from build123d import *

# Parameters (mm, degrees)
SKETCH1_W           = 40.1
SKETCH1_H           = 28.6
SKETCH1_W_2         = 36.5
SKETCH1_H_2         = 25
BOSS_EXTRUDE1_DEPTH = 8
SKETCH2_W           = 40.1
SKETCH2_H           = 28.6
SKETCH2_W_2         = 31
SKETCH2_H_2         = 23
BOSS_EXTRUDE2_DEPTH = 2
FILLET1_R           = 4
FILLET4_R           = 3
FILLET5_R           = 3
CUT_EXTRUDE1_REACH  = 45.732


with BuildPart() as part:
    # Sketch1 → Boss-Extrude1 (new body)
    with BuildSketch(Plane(origin=(0, 0, 0), x_dir=(1, 0, 0), z_dir=(0, 1, 0))):
        Rectangle(SKETCH1_W, SKETCH1_H)
        Rectangle(SKETCH1_W_2, SKETCH1_H_2, mode=Mode.SUBTRACT)
    extrude(amount=BOSS_EXTRUDE1_DEPTH)

    # Sketch2 → Boss-Extrude2 (add)
    with BuildSketch(Plane(origin=(0, 8, 0), x_dir=(1, 0, 0), z_dir=(0, 1, 0))):
        Rectangle(SKETCH2_W, SKETCH2_H)
        with Locations((-1.25, 0)):
            Rectangle(SKETCH2_W_2, SKETCH2_H_2, mode=Mode.SUBTRACT)
    extrude(amount=BOSS_EXTRUDE2_DEPTH)

    # Fillet1
    fillet1_edges = [part.edges().sort_by_distance(p)[0] for p in [
        (20.05, 5, 14.3),
        (-20.05, 5, 14.3),
        (-20.05, 5, -14.3),
        (20.05, 5, -14.3),
    ]]
    fillet(fillet1_edges, radius=FILLET1_R)

    # Fillet4
    # the kernel refuses this fillet: 3 mm, written as the material it takes off along each edge
    with BuildSketch(Plane(origin=(-20.05, 10, 10.3), x_dir=(1, 0, 0), z_dir=(0, 0, -1)), Plane(origin=(20.05, 10, -10.3), x_dir=(-1, 0, 0), z_dir=(0, 0, 1))) as fillet4_piece_1:
        with BuildLine():
            CenterArc((FILLET4_R, FILLET4_R), FILLET4_R, 180, 90)
            Line((0, FILLET4_R), (0, 0))
            Line((0, 0), (FILLET4_R, 0))
        make_face()
    extrude(amount=20.6, mode=Mode.SUBTRACT)
    with BuildSketch(Plane(origin=(-16.05, 10, -10.3), x_dir=(0, 0, -1), z_dir=(1, 0, 0))) as fillet4_piece_2:
        with BuildLine():
            CenterArc((4 - FILLET4_R, -FILLET4_R), FILLET4_R, 0, 90)
            Line((4, -FILLET4_R), (4, 0))
            Line((4, 0), (4 - FILLET4_R, 0))
        make_face()
    revolve(axis=Axis((-16.05, 10, -10.3), (0, 1, 0)), revolution_arc=90, mode=Mode.SUBTRACT)
    with BuildSketch(Plane(origin=(-16.05, 10, -14.3), x_dir=(0, 0, 1), z_dir=(1, 0, 0))) as fillet4_piece_3:
        with BuildLine():
            CenterArc((FILLET4_R, FILLET4_R), FILLET4_R, 180, 90)
            Line((0, FILLET4_R), (0, 0))
            Line((0, 0), (FILLET4_R, 0))
        make_face()
    extrude(amount=32.1, mode=Mode.SUBTRACT)
    with BuildSketch(Plane(origin=(16.05, 10, -10.3), x_dir=(0, 0, -1), z_dir=(-1, 0, 0))) as fillet4_piece_4:
        with BuildLine():
            CenterArc((4 - FILLET4_R, FILLET4_R), FILLET4_R, 270, 90)
            Line((4, FILLET4_R), (4, 0))
            Line((4, 0), (4 - FILLET4_R, 0))
        make_face()
    revolve(axis=Axis((16.05, 10, -10.3), (0, -1, 0)), revolution_arc=90, mode=Mode.SUBTRACT)
    with BuildSketch(Plane(origin=(16.05, 10, 10.3), x_dir=(0, 0, 1), z_dir=(-1, 0, 0))) as fillet4_piece_5:
        with BuildLine():
            CenterArc((4 - FILLET4_R, -FILLET4_R), FILLET4_R, 360, 90)
            Line((4, -FILLET4_R), (4, 0))
            Line((4, 0), (4 - FILLET4_R, 0))
        make_face()
    revolve(axis=Axis((16.05, 10, 10.3), (0, 1, 0)), revolution_arc=90, mode=Mode.SUBTRACT)
    with BuildSketch(Plane(origin=(16.05, 10, 14.3), x_dir=(0, -1, 0), z_dir=(-1, 0, 0))) as fillet4_piece_6:
        with BuildLine():
            CenterArc((FILLET4_R, -FILLET4_R), FILLET4_R, 90, 90)
            Line((0, -FILLET4_R), (0, 0))
            Line((0, 0), (FILLET4_R, 0))
        make_face()
    extrude(amount=32.1, mode=Mode.SUBTRACT)
    with BuildSketch(Plane(origin=(-16.05, 10, 10.3), x_dir=(0, 0, 1), z_dir=(1, 0, 0))) as fillet4_piece_7:
        with BuildLine():
            CenterArc((4 - FILLET4_R, FILLET4_R), FILLET4_R, 270, 90)
            Line((4, FILLET4_R), (4, 0))
            Line((4, 0), (4 - FILLET4_R, 0))
        make_face()
    revolve(axis=Axis((-16.05, 10, 10.3), (0, -1, 0)), revolution_arc=90, mode=Mode.SUBTRACT)

    # Fillet5
    # the kernel refuses this fillet: 3 mm, written as the material it adds along each edge
    with BuildSketch(Plane(origin=(-18.25, 8, 12.5), x_dir=(0, -1, 0), z_dir=(0, 0, -1))) as fillet5_piece_1_section:
        with BuildLine():
            CenterArc((FILLET5_R, -FILLET5_R), FILLET5_R, 90, 90)
            Line((0, -FILLET5_R), (0, 0))
            Line((0, 0), (FILLET5_R, 0))
        make_face()
    fillet5_piece_1 = extrude(amount=25, mode=Mode.PRIVATE)
    fillet5_piece_1 = split(fillet5_piece_1, bisect_by=Plane(origin=(-16.75, 7.23463982, 12), z_dir=(-1, 0, 0)), keep=Keep.TOP, mode=Mode.PRIVATE)
    fillet5_piece_1 = split(fillet5_piece_1, bisect_by=Plane(origin=(-17.756824707, 7.23463982, 11.5), z_dir=(0, 0, 1)), keep=Keep.TOP, mode=Mode.PRIVATE)
    add(fillet5_piece_1)
    with BuildSketch(Plane(origin=(-18.25, 8, 12.5), x_dir=(0, -1, 0), z_dir=(0, 0, -1))) as fillet5_piece_2_section:
        with BuildLine():
            CenterArc((FILLET5_R, -FILLET5_R), FILLET5_R, 90, 90)
            Line((0, -FILLET5_R), (0, 0))
            Line((0, 0), (FILLET5_R, 0))
        make_face()
    fillet5_piece_2 = extrude(amount=25, mode=Mode.PRIVATE)
    fillet5_piece_2 = split(fillet5_piece_2, bisect_by=Plane(origin=(-16.75, 7.927974855, 12), z_dir=(1, 0, 0)), keep=Keep.TOP, mode=Mode.PRIVATE)
    fillet5_piece_2 = split(fillet5_piece_2, bisect_by=Plane(origin=(-16.260247646, 7.927974855, 11.5), z_dir=(0, 0, 1)), keep=Keep.TOP, mode=Mode.PRIVATE)
    add(fillet5_piece_2)
    with BuildSketch(Plane(origin=(-18.25, 8, 12.5), x_dir=(0, -1, 0), z_dir=(0, 0, -1))) as fillet5_piece_3_section:
        with BuildLine():
            CenterArc((FILLET5_R, -FILLET5_R), FILLET5_R, 90, 90)
            Line((0, -FILLET5_R), (0, 0))
            Line((0, 0), (FILLET5_R, 0))
        make_face()
    fillet5_piece_3 = extrude(amount=25, mode=Mode.PRIVATE)
    fillet5_piece_3 = split(fillet5_piece_3, bisect_by=Plane(origin=(-16.75, 7.23463982, 0), z_dir=(-1, 0, 0)), keep=Keep.TOP, mode=Mode.PRIVATE)
    fillet5_piece_3 = split(fillet5_piece_3, bisect_by=Plane(origin=(-17.756824707, 7.23463982, 11.5), z_dir=(0, 0, -1)), keep=Keep.TOP, mode=Mode.PRIVATE)
    fillet5_piece_3 = split(fillet5_piece_3, bisect_by=Plane(origin=(-17.756824707, 7.23463982, -11.5), z_dir=(0, 0, 1)), keep=Keep.TOP, mode=Mode.PRIVATE)
    add(fillet5_piece_3)
    with BuildSketch(Plane(origin=(-18.25, 8, 12.5), x_dir=(0, -1, 0), z_dir=(0, 0, -1))) as fillet5_piece_4_section:
        with BuildLine():
            CenterArc((FILLET5_R, -FILLET5_R), FILLET5_R, 90, 90)
            Line((0, -FILLET5_R), (0, 0))
            Line((0, 0), (FILLET5_R, 0))
        make_face()
    fillet5_piece_4 = extrude(amount=25, mode=Mode.PRIVATE)
    fillet5_piece_4 = split(fillet5_piece_4, bisect_by=Plane(origin=(-16.75, 7.23463982, -12), z_dir=(-1, 0, 0)), keep=Keep.TOP, mode=Mode.PRIVATE)
    fillet5_piece_4 = split(fillet5_piece_4, bisect_by=Plane(origin=(-17.756824707, 7.23463982, -11.5), z_dir=(0, 0, -1)), keep=Keep.TOP, mode=Mode.PRIVATE)
    add(fillet5_piece_4)
    with BuildSketch(Plane(origin=(-18.25, 8, 12.5), x_dir=(0, -1, 0), z_dir=(0, 0, -1))) as fillet5_piece_5_section:
        with BuildLine():
            CenterArc((FILLET5_R, -FILLET5_R), FILLET5_R, 90, 90)
            Line((0, -FILLET5_R), (0, 0))
            Line((0, 0), (FILLET5_R, 0))
        make_face()
    fillet5_piece_5 = extrude(amount=25, mode=Mode.PRIVATE)
    fillet5_piece_5 = split(fillet5_piece_5, bisect_by=Plane(origin=(-16.75, 7.927974855, -12), z_dir=(1, 0, 0)), keep=Keep.TOP, mode=Mode.PRIVATE)
    fillet5_piece_5 = split(fillet5_piece_5, bisect_by=Plane(origin=(-16.260247646, 7.927974855, -11.5), z_dir=(0, 0, -1)), keep=Keep.TOP, mode=Mode.PRIVATE)
    add(fillet5_piece_5)
    with BuildSketch(Plane(origin=(18.25, 8, -12.5), x_dir=(0, -1, 0), z_dir=(0, 0, 1))) as fillet5_piece_6:
        with BuildLine():
            CenterArc((FILLET5_R, -FILLET5_R), FILLET5_R, 90, 90)
            Line((0, -FILLET5_R), (0, 0))
            Line((0, 0), (FILLET5_R, 0))
        make_face()
    extrude(amount=25)

    # Sketch3 → Cut-Extrude1 (cut, up to next)
    with BuildSketch(Plane(origin=(20.05, 0, 0), x_dir=(0, 0, -1), z_dir=(1, 0, 0)), mode=Mode.PRIVATE) as cut_extrude1_sk1:
        with BuildLine():
            Line((5.15, -1.5), (-5.15, -1.5))
            ThreePointArc((-5.15, -1.5), (-6.65, 0), (-5.15, 1.5))
            Line((-5.15, 1.5), (5.15, 1.5))
            ThreePointArc((5.15, 1.5), (6.65, 0), (5.15, -1.5))
        make_face()
    cut_extrude1_tool1 = extrude(cut_extrude1_sk1.sketch, amount=-CUT_EXTRUDE1_REACH, mode=Mode.PRIVATE) & part.part
    add(cut_extrude1_tool1.solids().sort_by_distance((20.05, 0, 0))[0], mode=Mode.SUBTRACT)


solid = part.part
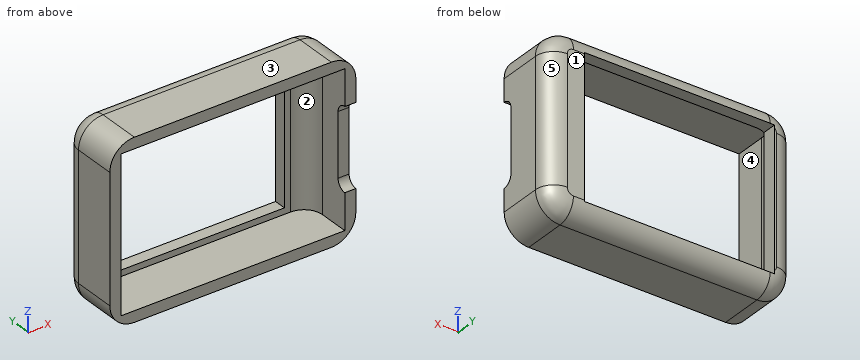
Geometry check sheet. Reference: the model listing, model coordinates, mm. Face numbers are marked on the shaded views. A direction names the side the tool comes from. Round coordinates to 2 decimals unless told otherwise and drop trailing zeros. Order: outer loops, then holes, each group sorted by start corner. A loop starts at its lowest first (then second) coordinate and runs counter-clockwise, first axis right, second up. Notation, with made-up numbers: M 70.5,88.5 L 86.5,88.5 A29 cw 86.5,115.5 Z; hole C 43.25,64 d7. An arc over 180 degrees is marked long. Answer in a Markdown table with one row per item.
(1) Sectioned sample at B-B, the plane x = -13. Record the cut outline in (y, z), and give its area (3 significant figures).
Responses:
| item | result |
|---|---|
| outline | M 0,-14.3 L 7,-14.3 A3 ccw 9.99,-11.5 L 8,-11.5 L 8,-12.5 L 0,-12.5 Z; M 0,12.5 L 8,12.5 L 8,11.5 L 9.99,11.5 A3 ccw 7,14.3 L 0,14.3 Z |
| area | 36.1 mm² |
(2) Sectioned sample at C-C, the plane y = 3.75. Record the cut outline in (x, z), and give its area (3 significant figures).
Responses:
| item | result |
|---|---|
| outline | M -20.05,-10.3 A4 ccw -16.05,-14.3 L 16.05,-14.3 A4 ccw 20.05,-10.3 L 20.05,10.3 A4 ccw 16.05,14.3 L -16.05,14.3 A4 ccw -20.05,10.3 Z; hole M -18.25,-12.5 L 18.25,-12.5 L 18.25,12.5 L -18.25,12.5 Z |
| area | 221 mm² |
(3) Tool access check on the marked faces 1 and 2. Record the directions out of +Z, -Z, +X, -X, +Y, -Y that give a thin tool (end or side, any length) a straight path to the whole face; none if there is none.
Responses:
| item | result |
|---|---|
| face 1 | +Z, -Z, +X, -X, +Y |
| face 2 | -Y |
(4) Sectioned sample at A-A, the plane z = -2.25. Record the cut outline in (x, y), and give its area (3 significant figures).
Responses:
| item | result |
|---|---|
| outline | M -20.05,0 L -18.25,0 L -18.25,5 A3 cw -16.75,7.6 L -16.75,10 L -17.05,10 A3 ccw -20.05,7 Z; M 14.25,8 L 15.25,8 A3 cw 18.25,5 L 18.25,1.5 L 20.05,1.5 L 20.05,7 A3 ccw 17.05,10 L 14.25,10 Z |
| area | 44.1 mm² |
(5) Sectioned sample at D-D, the plane z = -6. Record the cut outline in (x, y).
Responses:
| item | result |
|---|---|
| outline | M -20.05,0 L -18.25,0 L -18.25,5 A3 cw -16.75,7.6 L -16.75,10 L -17.05,10 A3 ccw -20.05,7 Z; M 14.25,8 L 15.25,8 A3 cw 18.25,5 L 18.25,1.24 L 20.05,1.24 L 20.05,7 A3 ccw 17.05,10 L 14.25,10 Z |
(6) Scan lines: probe 1 along Z at (x, y) = (10, 4); probe 2 along X at (y, z) = (2.5, 8); probe 3 along X at (y, z) = (6.5, -12.25). Record each from-to range of solid material in increasing order. Write a range as from..to.
Responses:
| item | result |
|---|---|
| probe 1 | z = -14.3..-12.5, 12.5..14.3 |
| probe 2 | x = -20.05..-18.25, 18.25..20.05 |
| probe 3 | x = -19.54..-17.85, 17.85..19.54 |
(7) Draft check along Z on the marked faces 3, 4 and 5. Enter one of: released by +Z, released by -Z, zero draft, split by the parting line, or undercut.
Responses:
| item | result |
|---|---|
| face 3 | released by +Z |
| face 4 | undercut |
| face 5 | zero draft |
(8) Go/stop test with flat-tipped pins: P1, Ø1.2, axis at y = 8.5, z = -4, coming from the +X side; P2, Ø1.6, axis at y = 9, z = 0, coming from the -X side; P3, Ø2, axis at x = 19, z = -2, coming from the -Y side; P4, Ø6, axis at x = -16, z = -6.5, coming from the +Y side. Record where each tip stops, or that it passes through.
Responses:
| item | result |
|---|---|
| P1 | stops at x = 19.91 |
| P2 | stops at x = -19.8 |
| P3 | stops at y = 1.5 |
| P4 | stops at y = 10 |
